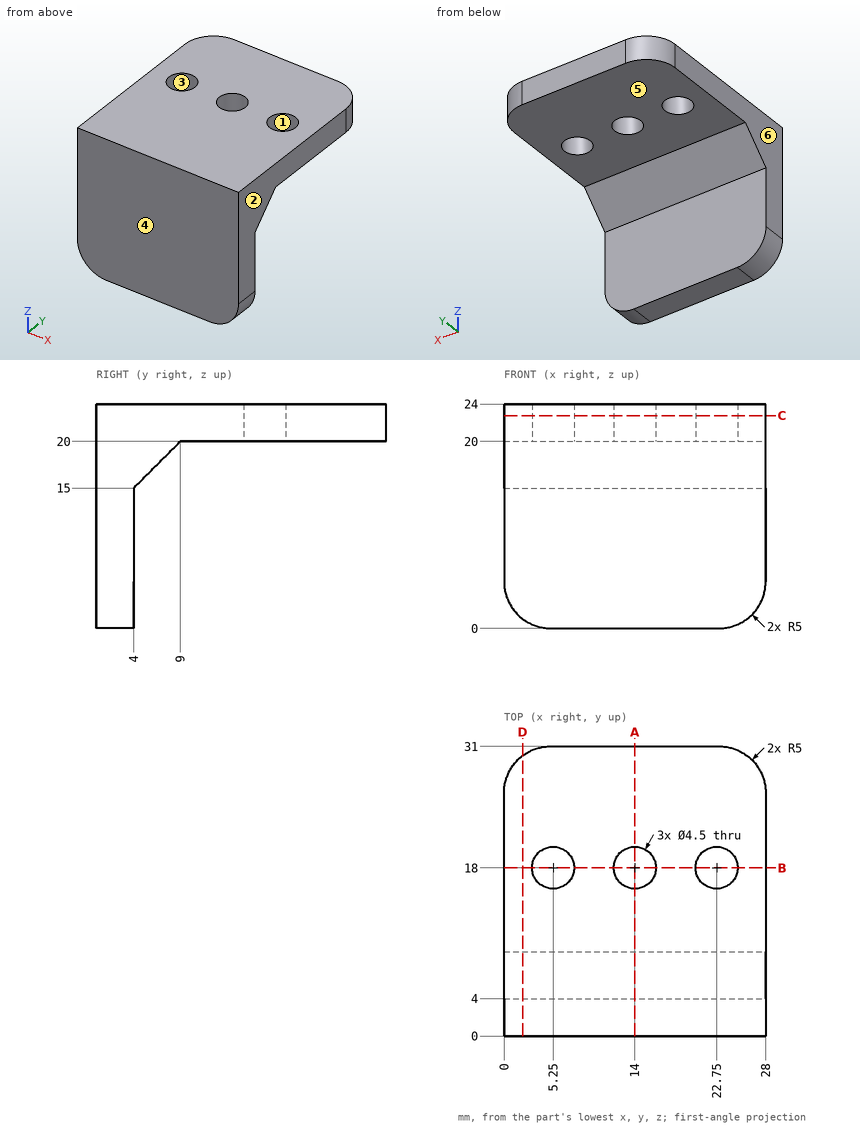
Study the drawing (mm; zero at the part's minimum x, y, z) and answer. A direction names the side the tool comes from. Give positions to 0.01 mm unless a question says otherwise; leave off trailing zeros. Write each loop counter-clockwise with the first axis right and the second up, starting at its lowest first coordinate (ties: lowest second). Pieces come first, ordered by that corner, then holes. Notation, with made-up numbers: (26.5, 71) - (46.5, 71) arc R8 ccw to (46.5, 82) - close; hole circle Ø7 at (5, -33.75). An arc over 180 degrees is marked (long way). Use a Markdown table: item, result.
1. A tool of negligible diameter and unlimited length cuts with its end or side. For the marked faces 5 and 6, from which of +Z, -Z, +X, -X, +Y, -Y can it reach the whole face along a straight path? Write none if from no direction.
Values follow:
| item | result |
|---|---|
| face 5 | -Z, +X, -X, +Y |
| face 6 | +Z, -Z, -X, +Y, -Y |
2. Each of these flat-tipped pins is pushed along its axis until it touches: P1, Ø12, axis at x = 6.5, z = 13.5, coming from the +Y side; P2, Ø1.5, axis at x = 3.5, y = 17, coming from the -Z side; P3, Ø4.5, axis at x = 19.5, z = 10.5, coming from the +Y side. Where does it stop, or does it pass through?
Values follow:
| item | result |
|---|---|
| P1 | stops at y = 8.5 |
| P2 | stops at z = 20 |
| P3 | stops at y = 4 |
3. Find the intervals of material crossed by probe 1 along X at (y, z) = (18, 21.65); probe 2 along Y at (x, z) = (22.75, 23); probe 3 along Z at (x, y) = (3.75, 14), in increasing order. Write a range as from..to.
Values follow:
| item | result |
|---|---|
| probe 1 | x = 0..3, 7.5..11.75, 16.25..20.5, 25..28 |
| probe 2 | y = 0..15.75, 20.25..31 |
| probe 3 | z = 20..24 |
4. Section A-A on x = 14 is taken. Write down the section's boundary in (y, z).
Values follow:
| item | result |
|---|---|
| outline | (0, 0) - (4, 0) - (4, 15) - (9, 20) - (15.75, 20) - (15.75, 24) - (0, 24) - close; (20.25, 20) - (31, 20) - (31, 24) - (20.25, 24) - close |
5. Section B-B on y = 18 is taken. Write down the section's boundary in (x, z).
Values follow:
| item | result |
|---|---|
| outline | (0, 20) - (3, 20) - (3, 24) - (0, 24) - close; (7.5, 20) - (11.75, 20) - (11.75, 24) - (7.5, 24) - close; (16.25, 20) - (20.5, 20) - (20.5, 24) - (16.25, 24) - close; (25, 20) - (28, 20) - (28, 24) - (25, 24) - close |
6. Section D-D on x = 2 is taken. Write down the section's boundary in (y, z).
Values follow:
| item | result |
|---|---|
| outline | (0, 1) - (4, 1) - (4, 15) - (9, 20) - (30, 20) - (30, 24) - (0, 24) - close |
7. Section C-C on z = 22.75 is taken. Write down the section's boundary in (x, y), plus the area to 3 significant figures.
Values follow:
| item | result |
|---|---|
| outline | (0, 0) - (28, 0) - (28, 26) arc R5 ccw to (23, 31) - (5, 31) arc R5 ccw to (0, 26) - close; hole circle Ø4.5 at (5.25, 18); hole circle Ø4.5 at (14, 18); hole circle Ø4.5 at (22.75, 18) |
| area | 810 mm² |
8. For a pull along X with two mould halves and no side action, classify the marked faces 1, 2, 3 and 4 as released by +X, released by -X, zero draft, split by the parting line, or undercut.
Values follow:
| item | result |
|---|---|
| face 1 | undercut |
| face 2 | released by +X |
| face 3 | undercut |
| face 4 | zero draft |
